Autodesk Inventor part; units mm, degrees
ref_plane "Work Plane1" through (-7.2255, 0, 0) normal (0, 0, -1) x (1, 0, 0)
ref_plane "YZ Plane" through (0, 0, 0) normal (1, 0, 0) x (0, 1, 0)
ref_plane "XZ Plane" through (0, 0, 0) normal (0, 1, 0) x (-1, 0, 0)
sketch "Sketch1" plane through (0, 0, 0) normal (1, 0, 0) x (0, 1, 0)
  line L0 (1.7321, -3) -> (-1.7321, -3)
  line L1 (-1.7321, -3) -> (-3.4641, 0)
  line L2 (-3.4641, 0) -> (-1.7321, 3)
  line L3 (-1.7321, 3) -> (1.7321, 3)
  line L4 (1.7321, 3) -> (3.4641, 0)
  line L5 (3.4641, 0) -> (1.7321, -3)
  point P0 (0, 0)
  point P1 (0, 0)
  dimension "d0" = 6.9282
extrude "Body" add sketch "Sketch1" along normal blind 2.2
sketch "Sketch2" plane through (2.2, 0, 0) normal (1, 0, 0) x (0, 0, -1)
  point P0 (0, 0)
hole "Thread" at (2.2, 0, 0) direction (-1, 0, 0) diameter 2.85 end through all
chamfer "Chamfer2" distance 0.3248 angle 30 1 edges at (2.2, 0, 1.425) measured on face at (2.2, -2.123, -1.2698)
chamfer "Chamfer1" distance 0.3248 angle 30 1 edges at (0, 0, 1.425) measured on face at (0, -2.123, -1.2698)
ref_plane "Work Plane1" through (-7.2255, 0, 0) normal (0, 0, -1) x (1, 0, 0)
equation "\"d0\" = 1.1547 * SW"
equation "\"d1\" = KOH"
equation "\"d12\" = -0.5 * GD1 + 0.5 * NND"
equation "\"d19\" = -0.5 * GD1 + 0.5 * NND"
equation "\"d10\" = -0.5 * GD1 + 0.5 * NND"
equation "\"d18\" = -0.5 * GD1 + 0.5 * NND"
equation "\"NND\" = 3.5"
equation "\"KOH\" = 2.2"
equation "\"SW\" = 6"
equation "\"GUL\" = 0.541266 * PTC"
equation "\"THREADDIA\" = 3.5"
equation "\"TOA\" = 30deg"
equation "\"PTC\" = 0.6"
equation "\"E0\" = 1.155 * SW"
equation "\"GAL\" = 0.541266 * PTC"
properties part number "AS 1474 - M3.5" material "Steel, Mild"
Source: CAD feature listing. Evaluate the final solid. Frame: model axes, mm. Round coordinates to 2 decimals unless told otherwise and drop trailing zeros. Loops run counter-clockwise (first coordinate to the right, second up) from the corner with the lowest first, then second, coordinate; pieces in that order, holes last. Notation, with made-up numbers: M 86,27.25 L 130,27.25 A16 cw 130,42.25 Z; hole C 42,42 d4. An arc over 180 degrees is marked long. Use a Markdown table: item, result. Add a question column.
1. Contact query for a flat-ended pin moving along its axis: pin 1 (2.5 mm diameter, centred on y = 0, z = 0, fed in from +X). Output: stop coordinate, or through.
2. Cut plane D-D, the plane z = -2.3. Output: boundary loops of the cut face in (x, y).
3. Ray query, line 1 along Z through (x, y) = (1.45, 0) (3 decimals); line 2 along Z through (x, y) = (0.7, 1.25); line 3 along Y through (x, z) = (1.4, 2.4). Return the intervals inside material, ascending. Write a range as [from, to].
4. Cut plane B-B, the plane x = 1.65. Output: boundary loops of the cut face in (y, z) (3 decimals).
5. Cut plane C-C, the plane y = -2.5. Output: boundary loops of the cut face in (x, z).
6. Cut plane A-A, the plane y = 0. Output: boundary loops of the cut face in (x, z) (3 decimals), and give its area (3 significant figures).
7. Pull-direction query (Y, two-part tool) for faces 1 (the cylindrical face through (1.09, 0.87, 1.13)), 2 (the flat face through (1.1, -2.6, 1.5)), 3 (the flat face through (1, 0, 3)), 4 (the flat face through (1.1, 2.6, -1.5)); classes: +Y half, -Y half, draft (parallel to the pull), parting line (faces both ways), or undercut.
Solution:
| question | item | result |
|---|---|---|
| 1 | pin 1 | passes through |
| 2 | outline | M 0,-2.14 L 2.2,-2.14 L 2.2,2.14 L 0,2.14 Z |
| 3 | line 1 | z = [-3, -1.425], [1.425, 3] |
| 3 | line 2 | z = [-3, -0.68], [0.68, 3] |
| 3 | line 3 | y = [-2.08, 2.08] |
| 4 | outline | M -3.464,0 L -1.732,-3 L 1.732,-3 L 3.464,0 L 1.732,3 L -1.732,3 Z; hole C 0,0 d2.85 |
| 5 | outline | M 0,-1.67 L 2.2,-1.67 L 2.2,1.67 L 0,1.67 Z |
| 6 | outline | M 0,-3 L 2.2,-3 L 2.2,-1.75 L 2.012,-1.425 L 0.188,-1.425 L 0,-1.75 Z; M 0,1.75 L 0.188,1.425 L 2.012,1.425 L 2.2,1.75 L 2.2,3 L 0,3 Z |
| 6 | area | 6.81 mm2 |
| 7 | face 1 | undercut |
| 7 | face 2 | -Y half |
| 7 | face 3 | draft |
| 7 | face 4 | +Y half |
